```python
from build123d import *

# Parameters (mm, degrees)
SKETCH1_W           = 52.324
SKETCH1_H           = 160.02
BOSS_EXTRUDE1_DEPTH = 5.334
SKETCH2_W           = 5.334
SKETCH2_H           = 22.86
CUT_EXTRUDE1_DEPTH  = 115.417820658
SKETCH3_W           = 5.334
SKETCH3_H           = 38.1
BOSS_EXTRUDE2_DEPTH = 50.8
SKETCH4_W           = 23.876
SKETCH4_H           = 12.192
CUT_EXTRUDE2_DEPTH  = 151.047185381
SKETCH5_W           = 19.05
SKETCH5_H           = 6.35
CUT_EXTRUDE3_DEPTH  = 151.047185381
SKETCH6_W           = 5.334
SKETCH6_H           = 12.7
BOSS_EXTRUDE3_DEPTH = 25.4
SKETCH7_W           = 5.334
SKETCH7_H           = 12.7
BOSS_EXTRUDE4_DEPTH = 25.4
SKETCH8_W           = 5.334
SKETCH8_H           = 14.2875
CUT_EXTRUDE4_DEPTH  = 151.047185381
SKETCH9_W           = 5.334
SKETCH9_H           = 12.7
CUT_EXTRUDE5_DEPTH  = 151.047185381
CUT_EXTRUDE6_DEPTH  = 151.047185381
SKETCH11_W          = 5.334
SKETCH11_H          = 22.86
BOSS_EXTRUDE5_DEPTH = 8.89
SKETCH12_W          = 5.334
SKETCH12_H          = 7.62
CUT_EXTRUDE7_DEPTH  = 151.047185381


with BuildPart() as part:
    # Sketch1 → Boss-Extrude1 (new body)
    with BuildSketch(Plane.XY):
        with Locations((-41.181308627, -12.336439624)):
            Rectangle(SKETCH1_W, SKETCH1_H)
    extrude(amount=BOSS_EXTRUDE1_DEPTH)

    # Sketch2 → Cut-Extrude1 (cut, through all)
    with BuildSketch(Plane.XY.offset(5.334)):
        with Locations((-17.686308627, 56.243560376)):
            Rectangle(SKETCH2_W, SKETCH2_H)
        with Locations((-17.686308627, 10.523560376)):
            Rectangle(SKETCH2_W, SKETCH2_H)
        with Locations((-17.686308627, -35.196439624)):
            Rectangle(SKETCH2_W, SKETCH2_H)
        with Locations((-17.686308627, -80.916439624)):
            Rectangle(SKETCH2_W, SKETCH2_H)
    extrude(amount=-CUT_EXTRUDE1_DEPTH, mode=Mode.SUBTRACT)

    # Sketch3 → Boss-Extrude2 (add)
    with BuildSketch(Plane.ZY.offset(67.343308627)):
        with Locations((2.667, 2.903560376)):
            Rectangle(SKETCH3_W, SKETCH3_H)
    extrude(amount=BOSS_EXTRUDE2_DEPTH)

    # Sketch4 → Cut-Extrude2 (cut, through all)
    with BuildSketch(Plane.XY.offset(5.334)):
        with Locations((-92.997308627, 2.903560376)):
            Rectangle(SKETCH4_W, SKETCH4_H)
    extrude(amount=-CUT_EXTRUDE2_DEPTH, mode=Mode.SUBTRACT)

    # Sketch5 → Cut-Extrude3 (cut, through all)
    with BuildSketch(Plane.XY.offset(5.334)):
        with Locations((-57.818308627, 25.128560376)):
            Rectangle(SKETCH5_W, SKETCH5_H)
        with Locations((-57.818308627, -19.321439624)):
            Rectangle(SKETCH5_W, SKETCH5_H)
    extrude(amount=-CUT_EXTRUDE3_DEPTH, mode=Mode.SUBTRACT)

    # Sketch6 → Boss-Extrude3 (add)
    with BuildSketch(Plane.ZY.offset(67.343308627)):
        with Locations((2.667, 34.653560376)):
            Rectangle(SKETCH6_W, SKETCH6_H)
    extrude(amount=BOSS_EXTRUDE3_DEPTH)

    # Sketch7 → Boss-Extrude4 (add)
    with BuildSketch(Plane.ZY.offset(67.343308627)):
        with Locations((2.667, -28.846439624)):
            Rectangle(SKETCH7_W, SKETCH7_H)
    extrude(amount=BOSS_EXTRUDE4_DEPTH)

    # Sketch8 → Cut-Extrude4 (cut, through all)
    with BuildSketch(Plane.XY.offset(5.334)):
        with Locations((-64.676308627, -42.340189624)):
            Rectangle(SKETCH8_W, SKETCH8_H)
        with Locations((-64.676308627, -70.915189624)):
            Rectangle(SKETCH8_W, SKETCH8_H)
    extrude(amount=-CUT_EXTRUDE4_DEPTH, mode=Mode.SUBTRACT)

    # Sketch9 → Cut-Extrude5 (cut, through all)
    with BuildSketch(Plane.XY.offset(5.334)):
        with Locations((-64.676308627, 2.649560376)):
            Rectangle(SKETCH9_W, SKETCH9_H)
    extrude(amount=-CUT_EXTRUDE5_DEPTH, mode=Mode.SUBTRACT)

    # Sketch10 → Cut-Extrude6 (cut, through all)
    with BuildSketch(Plane.XY.offset(5.334)):
        Polygon((-57.379441561, -80.781874862), (-46.432343901, -87.220124068), (-44.50086914, -83.93599477), (-55.447966799, -77.497745564), align=None)
        Polygon((-45.287966799, -77.497745564), (-34.34086914, -83.93599477), (-36.272343901, -87.220124068), (-47.219441561, -80.781874862), align=None)
        Polygon((-35.127966799, -77.497745564), (-24.18086914, -83.93599477), (-26.112343901, -87.220124068), (-37.059441561, -80.781874862), align=None)
    extrude(amount=-CUT_EXTRUDE6_DEPTH, mode=Mode.SUBTRACT)

    # Sketch11 → Boss-Extrude5 (add)
    with BuildSketch(Plane(origin=(-15.019308627, 0, 0), x_dir=(0, 0, -1), z_dir=(1, 0, 0))):
        with Locations((-2.667, 33.383560376)):
            Rectangle(SKETCH11_W, SKETCH11_H)
    extrude(amount=BOSS_EXTRUDE5_DEPTH)

    # Sketch12 → Cut-Extrude7 (cut, through all)
    with BuildSketch(Plane.XY.offset(5.334)):
        with Locations((-12.352308627, 33.383560376)):
            Rectangle(SKETCH12_W, SKETCH12_H)
    extrude(amount=-CUT_EXTRUDE7_DEPTH, mode=Mode.SUBTRACT)


solid = part.part
```
Part model, mm, in its own coordinate system. A direction names the side the tool comes from. Give positions to 0.01 mm unless a question says otherwise; leave off trailing zeros. Order: outer loops, then holes, each group sorted by start corner. A loop starts at its lowest first (then second) coordinate and runs counter-clockwise, first axis right, second up. Notation, with made-up numbers: M -39,16 L -24,16 A12 cw -24,32 Z; hole C 13.5,5.25 d11. An arc over 180 degrees is marked long. Use a Markdown table: item, result. Add a question column.
(1) Mould opens along X. For faces 1 (the face through (-65, -63.771, 3)), 2 (the face through (-39.891, -80.672, 2.704)), 3 (the face through (-67.343, 54, 3)) say: +X half, -X half, draft (parallel to the pull), parting line (faces both ways), or undercut.
(2) Saw through at C-C, the plane z = 1.2. Give the number of separate pieces and of enclosed holes in the cut face, and give its area (3 significant figures).
(3) Saw through at B-B, the plane y = 4.5. Give the cut face in (x, z), and give its area (3 significant figures).
(4) Saw through at D-D, the plane x = -109.5. Give the cut face in (y, z).
(5) Saw through at A-A, the plane x = -60. Give the cut face in (y, z), and give its area (3 significant figures).
(6) Probe line 1 along Y through (x, z) = (-89, 3.8); line 2 along X through (y, z) = (7, 3.25); line 3 along Y through (x, z) = (-74.5, 0.95). List the from-to ranges inside material, lowest first. Write a range as [from, to].
(7) Drop flat-ended pins along their axis: P1, Ø1.5, axis at x = -93, z = 1.5, coming from the -Y side; P2, Ø1.5, axis at y = -46.5, z = 1.5, coming from the -X side; P3, Ø3, axis at y = -56.5, z = 3.5, coming from the -X side. Give the stop position or say it passes through.
(8) 3-axis set-ups, long thin cutter, end or side, ignore diameter. For faces 4 (the face through (-84, -16.146, 3)), 5 (the face through (-20.353, -81, 3)), 6 (the face through (-31.509, -84.046, 2.704)), 7 (the face through (-18, -0.906, 3)): which of +Z, -Z, +X, -X, +Y, -Y reach the whole face in a straight line?
Answer key:
| question | item | result |
|---|---|---|
| 1 | face 1 | draft |
| 1 | face 2 | undercut |
| 1 | face 3 | -X half |
| 2 | separate pieces | 1 |
| 2 | enclosed holes | 6 |
| 2 | area | 9,730 mm^2 |
| 3 | outline | M -118.14,0 L -104.94,0 L -104.94,5.33 L -118.14,5.33 Z; M -81.06,0 L -67.34,0 L -67.34,5.33 L -81.06,5.33 Z; M -62.01,0 L -20.35,0 L -20.35,5.33 L -62.01,5.33 Z |
| 3 | area | 366 mm^2 |
| 4 | outline | M -16.15,0 L 21.95,0 L 21.95,5.33 L -16.15,5.33 Z |
| 5 | outline | M -92.35,0 L -22.5,0 L -22.5,5.33 L -92.35,5.33 Z; M -16.15,0 L 21.95,0 L 21.95,5.33 L -16.15,5.33 Z; M 28.3,0 L 67.67,0 L 67.67,5.33 L 28.3,5.33 Z |
| 5 | area | 786 mm^2 |
| 6 | line 1 | [-35.2, -22.5], [-16.15, -3.19], [9, 21.95], [28.3, 41] |
| 6 | line 2 | [-118.14, -104.94], [-81.06, -67.34], [-62.01, -20.35] |
| 6 | line 3 | [-35.2, -22.5], [-16.15, 21.95], [28.3, 41] |
| 7 | P1 | y = -35.2 |
| 7 | P2 | x = -62.01 |
| 7 | P3 | x = -67.34 |
| 8 | face 4 | +Z, -Z, -X |
| 8 | face 5 | +Z, -Z, +X, -Y |
| 8 | face 6 | +Z, -Z |
| 8 | face 7 | +Z, -Z, +X |
